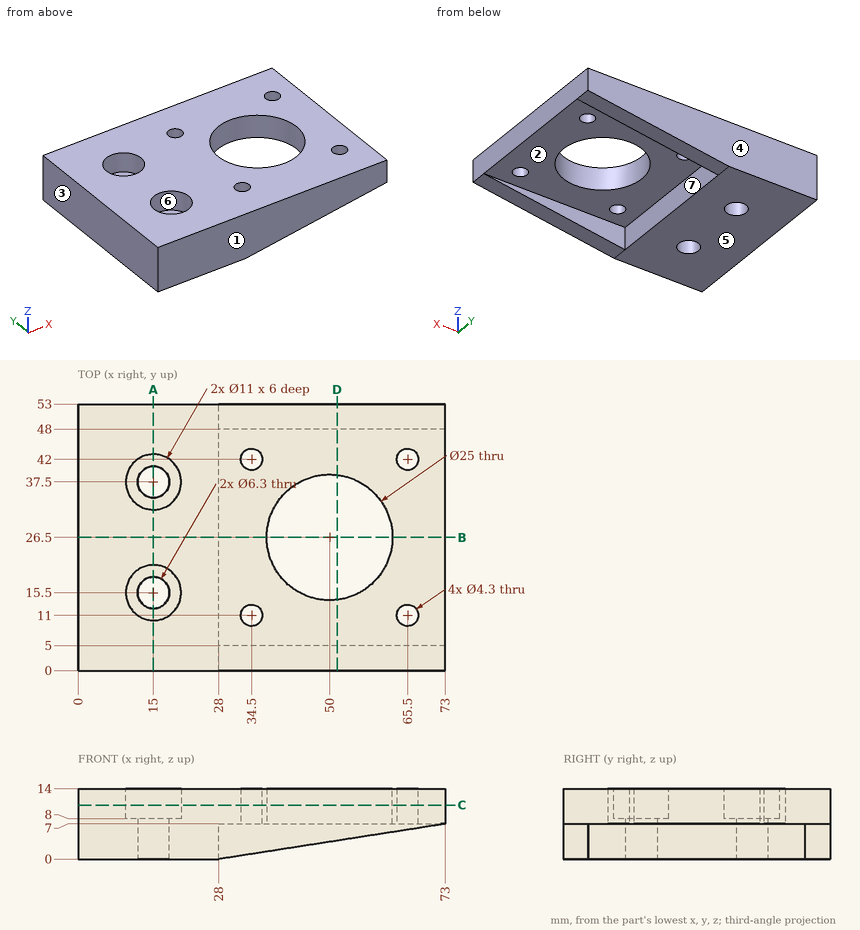
The drawing under review shows one solid part. Ordinate dimensions are in mm from its lowest x, y, z. A direction names the side the tool comes from. Round coordinates to 2 decimals unless told otherwise and drop trailing zeros. Write each loop counter-clockwise with the first axis right and the second up, starting at its lowest first coordinate (ties: lowest second). Pieces come first, ordered by that corner, then holes. Notation, with made-up numbers: (56.5, 1) - (78.5, 1) arc R31 cw to (78.5, 40) - close; hole circle Ø4 at (64.5, 5). An arc over 180 degrees is marked (long way). Use a Markdown table: item, result. Add a question column.
1. We need section B-B (y = 26.5). State the section outline as (x, z) points.
2. Wall thickness on probe 1 along Y at (x, z) = (34.5, 10.5); probe 2 along Y at (x, z) = (15, 11.35); probe 3 along X at (y, z) = (37.5, 6): over which ranges is each line inside the solid? List them lowest first.
3. We need section C-C (z = 10.75). State the section outline as (x, y) points.
4. For the marked faces 5, 6 and 7, list the 3-axis set-ups (+Z, -Z, +X, -X, +Y, -Y) from which the entire face can be reached by the end or side of a thin tool; tool diameter is ignored.
5. Mouldability with a two-part tool opening along Y and no side actions: class the marked faces 1, 2, 3 and 4 as +Y half, -Y half, draft (parallel to the pull), parting line (faces both ways), or undercut.
6. We need section A-A (x = 15). State the section outline as (y, z) points, then the cut area to 3 significant figures.
7. Clearance check with flat-ended pins moving along their axes: pin 1 (4 mm diameter, centred on x = 34.5, y = 11, fed in from +Z); pin 2 (10 mm diameter, centred on x = 34, y = 33, fed in from -Z); pin 3 (2 mm diameter, centred on y = 17.5, z = 4.5, fed in from +X); pin 4 (10 mm diameter, centred on x = 15, y = 37.5, fed in from +Z). State where each tip first meets the part, or that it passes through.
8. We need section D-D (x = 51.5). State the section outline as (y, z) points.
Output:
| question | item | result |
|---|---|---|
| 1 | outline | (0, 0) - (28, 0) - (28, 7) - (37.5, 7) - (37.5, 14) - (0, 14) - close; (62.5, 7) - (73, 7) - (73, 14) - (62.5, 14) - close |
| 2 | probe 1 | y = 0 to 8.85, 13.15 to 39.85, 44.15 to 53 |
| 2 | probe 2 | y = 0 to 10, 21 to 32, 43 to 53 |
| 2 | probe 3 | x = 0 to 11.85, 18.15 to 28 |
| 3 | outline | (0, 0) - (73, 0) - (73, 53) - (0, 53) - close; hole circle Ø11 at (15, 15.5); hole circle Ø11 at (15, 37.5); hole circle Ø4.3 at (34.5, 11); hole circle Ø4.3 at (34.5, 42); hole circle Ø25 at (50, 26.5); hole circle Ø4.3 at (65.5, 11); hole circle Ø4.3 at (65.5, 42) |
| 4 | face 5 | -Z, +X, -X, +Y, -Y |
| 4 | face 6 | +Z |
| 4 | face 7 | -Z, +X |
| 5 | face 1 | -Y half |
| 5 | face 2 | undercut |
| 5 | face 3 | draft |
| 5 | face 4 | +Y half |
| 6 | outline | (0, 0) - (12.35, 0) - (12.35, 8) - (10, 8) - (10, 14) - (0, 14) - close; (18.65, 0) - (34.35, 0) - (34.35, 8) - (32, 8) - (32, 14) - (21, 14) - (21, 8) - (18.65, 8) - close; (40.65, 0) - (53, 0) - (53, 14) - (43, 14) - (43, 8) - (40.65, 8) - close |
| 6 | area | 509 mm2 |
| 7 | pin 1 | passes through |
| 7 | pin 2 | stops at z = 7 |
| 7 | pin 3 | stops at x = 28 |
| 7 | pin 4 | stops at z = 8 |
| 8 | outline | (0, 3.66) - (5, 3.66) - (5, 7) - (14.09, 7) - (14.09, 14) - (0, 14) - close; (38.91, 7) - (48, 7) - (48, 3.66) - (53, 3.66) - (53, 14) - (38.91, 14) - close |
